from build123d import *

# Parameters (mm, degrees)
SKETCH_1_R               = 80
EXTRUDE_1_DEPTH          = 60
SKETCH_2_R               = 65
EXTRUDE_2_DEPTH          = 40
SKETCH_3_R               = 70
CUT_EXTRUDE_1_DEPTH      = 40
SKETCH_4_R               = 50
CUT_EXTRUDE_2_DEPTH      = 151.996688705
CHAMFER_1_SIZE           = 1
CUT_EXTRUDE_3_DEPTH      = 151.996688705
CUT_EXTRUDE_3_DEPTH_BACK = 151.996688705
SKETCH_5_R               = 10
CHAMFER_2_SIZE           = 5


with BuildPart() as part:
    # Эскиз1 → Бобышка-Вытянуть1 (new body)
    with BuildSketch(Plane.XY):
        Circle(SKETCH_1_R)
    extrude(amount=EXTRUDE_1_DEPTH)

    # Эскиз2 → Бобышка-Вытянуть2 (add)
    with BuildSketch(Plane.XY.offset(60)):
        Circle(SKETCH_2_R)
    extrude(amount=EXTRUDE_2_DEPTH)

    # Эскиз3 → Вырез-Вытянуть1 (cut)
    with BuildSketch(Plane(origin=(0, 0, 0), x_dir=(-1, 0, 0), z_dir=(0, 0, -1))):
        Circle(SKETCH_3_R)
    extrude(amount=-CUT_EXTRUDE_1_DEPTH, mode=Mode.SUBTRACT)

    # Эскиз4 → Вырез-Вытянуть2 (cut, through all)
    with BuildSketch(Plane.XY.offset(100)):
        Circle(SKETCH_4_R)
    extrude(amount=-CUT_EXTRUDE_2_DEPTH, mode=Mode.SUBTRACT)

    # Фаска1
    chamfer_1_edges = [part.edges().sort_by_distance(p)[0] for p in [
        (70, 0, 0),
        (-80, 0, 0),
    ]]
    chamfer(chamfer_1_edges, length=CHAMFER_1_SIZE)

    # Эскиз5 → Вырез-Вытянуть3 (cut, two sides: drawn at the far end of the back side and taken through both)
    with BuildSketch(Plane(origin=(0, 0, 0), x_dir=(0, 0, -1), z_dir=(1, 0, 0)).offset(-CUT_EXTRUDE_3_DEPTH_BACK)):
        with Locations((-75, 0)):
            Circle(SKETCH_5_R)
    extrude(amount=CUT_EXTRUDE_3_DEPTH + CUT_EXTRUDE_3_DEPTH_BACK, mode=Mode.SUBTRACT)

    # Фаска2
    chamfer_2_edges = [part.edges().sort_by_distance(p)[0] for p in [
        (-50, 0, 100),
    ]]
    chamfer(chamfer_2_edges, length=CHAMFER_2_SIZE)


solid = part.part
Can you work these out from the model? Positions are in its coordinate system, mm. A direction names the side the tool comes from. Round coordinates to 2 decimals unless told otherwise and drop trailing zeros. Write each loop counter-clockwise with the first axis right and the second up, starting at its lowest first coordinate (ties: lowest second). Pieces come first, ordered by that corner, then holes. Notation, with made-up numbers: (19, 88) - (71, 88) arc R31 cw to (71, 121) - close; hole circle Ø11 at (35, -37). An arc over 180 degrees is marked (long way). Write each question's results on one line, items separated by ' | '. Start each with the question number.
1) For pin 1 Ø4 at (x, y) = (-40.5, -46.5) entering from -Z; pin 2 Ø4 at (x, z) = (29.5, 35.5) entering from -Y; pin 3 Ø10 at (y, z) = (-37, 31) entering from -X; pin 4 Ø18 at (y, z) = (0, 75) entering from -X, each with a flat end and sliding along its axis, tell me the tip position at first contact or that it passes through.
2) Suppose I cut it at D-D (z = 37). List the corners of the cut face in (x, y) for me.
3) We'd pull the mould along Y, two halves only. Please class faces 4 (the cylindrical face through (62, 19.52, 79.72)), 5 (the cylindrical face through (47.69, 15.02, 67.89)), 6 (the flat face through (-53.3, 14.7, 100)): released by +Y, released by -Y, zero draft, split by the parting line, or undercut.
4) Suppose I cut it at B-B (x = 0). List the corners of the cut face in (y, z) for me.
5) Suppose I cut it at A-A (y = 0). Give the number of separate pieces and of enclosed holes in the cut face, and give its area (3 significant figures).
6) Suppose I cut it at C-C (z = 75). List the corners of the cut face in (x, y) for me.
7) Please list where these lines run through material, in increasing order: line 1 (Z direction, x = 61.75, y = 0); line 2 (Y direction, x = 0, z = 9); line 3 (Y direction, x = -15, z = 39.5).
8) Which directions (+Z, -Z, +X, -X, +Y, -Y) give clear straight access to the entire face, cutting with the end or side of a thin tool? Please do faces 1 (the flat face through (48, 17, 40)), 2 (the flat face through (-65, 30, 0)), 3 (the flat face through (0, 66, 60)).
Here are the results:
1) pin 1: stops at z = 40 | pin 2: stops at y = -75.12 | pin 3: stops at x = -73.32 | pin 4: passes through
2) outline: circle Ø160 at (0, 0); hole circle Ø140 at (0, 0)
3) face 4: split by the parting line | face 5: undercut | face 6: zero draft
4) outline: (-80, 1) - (-79, 0) - (-71, 0) - (-70, 1) - (-70, 40) - (-50, 40) - (-50, 95) - (-55, 100) - (-65, 100) - (-65, 60) - (-80, 60) - close; (50, 40) - (70, 40) - (70, 1) - (71, 0) - (79, 0) - (80, 1) - (80, 60) - (65, 60) - (65, 100) - (55, 100) - (50, 95) - close
5) separate pieces: 4 | enclosed holes: 0 | area: 2,570 mm2
6) outline: (-64.23, -10) arc R65 ccw to (64.23, -10) - (48.99, -10) arc R50 cw to (-48.99, -10) - close; (-64.23, 10) - (-48.99, 10) arc R50 cw to (48.99, 10) - (64.23, 10) arc R65 ccw to start
7) line 1: z = 40 to 65, 85 to 100 | line 2: y = -80 to -70, 70 to 80 | line 3: y = -78.58 to -68.37, 68.37 to 78.58
8) face 1: -Z | face 2: -Z, +X, -X, +Y, -Y | face 3: +Z
